from build123d import *

# Parameters (mm, degrees)
F1_DEPTH = 2.25
F2_R     = 0.375
F3_DEPTH = 2.251


with BuildPart() as f1:
    # F0 (on Top) → F1 (new body)
    with BuildSketch(Plane.XY):
        with BuildLine():
            Line((3.396481, 0.154959), (3.496284, 0.161238))
            ThreePointArc((3.496284, 0.161238), (3.474149, 0.424604), (3.432204, 0.685549))
            Line((3.432204, 0.685549), (3.359394, 0.661892))
            Line((3.359394, 0.661892), (3.251238, 0.994762))
            Line((3.251238, 0.994762), (3.346343, 1.025663))
            ThreePointArc((3.346343, 1.025663), (3.259407, 1.27525), (3.153886, 1.517566))
            Line((3.153886, 1.517566), (3.089246, 1.476545))
            Line((3.089246, 1.476545), (2.901707, 1.772059))
            Line((2.901707, 1.772059), (2.98614, 1.825642))
            ThreePointArc((2.98614, 1.825642), (2.839865, 2.045768), (2.677397, 2.254228))
            Line((2.677397, 2.254228), (2.62499, 2.198421))
            Line((2.62499, 2.198421), (2.369851, 2.438012))
            Line((2.369851, 2.438012), (2.438306, 2.510909))
            ThreePointArc((2.438306, 2.510909), (2.241884, 2.687742), (2.032678, 2.849249))
            Line((2.032678, 2.849249), (1.995797, 2.782162))
            Line((1.995797, 2.782162), (1.689089, 2.950775))
            Line((1.689089, 2.950775), (1.737265, 3.038406))
            ThreePointArc((1.737265, 3.038406), (1.503037, 3.160835), (1.260238, 3.265241))
            Line((1.260238, 3.265241), (1.241199, 3.191089))
            Line((1.241199, 3.191089), (0.902195, 3.278131))
            Line((0.902195, 3.278131), (0.927064, 3.374989))
            ThreePointArc((0.927064, 3.374989), (0.669748, 3.435322), (0.408613, 3.476066))
            Line((0.408613, 3.476066), (0.408613, 3.399509))
            Line((0.408613, 3.399509), (0.058613, 3.399509))
            Line((0.058613, 3.399509), (0.058613, 3.499509))
            ThreePointArc((0.058613, 3.499509), (-0.205623, 3.493955), (-0.468687, 3.468477))
            Line((-0.468687, 3.468477), (-0.449648, 3.394325))
            Line((-0.449648, 3.394325), (-0.788652, 3.307284))
            Line((-0.788652, 3.307284), (-0.813521, 3.404142))
            ThreePointArc((-0.813521, 3.404142), (-1.068074, 3.333049), (-1.316537, 3.242951))
            Line((-1.316537, 3.242951), (-1.279656, 3.175864))
            Line((-1.279656, 3.175864), (-1.586363, 3.00725))
            Line((-1.586363, 3.00725), (-1.634538, 3.09488))
            ThreePointArc((-1.634538, 3.09488), (-1.863414, 2.962716), (-2.081665, 2.813658))
            Line((-2.081665, 2.813658), (-2.029258, 2.757851))
            Line((-2.029258, 2.757851), (-2.284397, 2.518259))
            Line((-2.284397, 2.518259), (-2.352852, 2.591156))
            ThreePointArc((-2.352852, 2.591156), (-2.541669, 2.406225), (-2.715994, 2.207573))
            Line((-2.715994, 2.207573), (-2.651355, 2.166552))
            Line((-2.651355, 2.166552), (-2.838894, 1.871037))
            Line((-2.838894, 1.871037), (-2.923327, 1.92462))
            ThreePointArc((-2.923327, 1.92462), (-3.060222, 1.698541), (-3.179667, 1.462778))
            Line((-3.179667, 1.462778), (-3.106857, 1.43912))
            Line((-3.106857, 1.43912), (-3.215013, 1.106251))
            Line((-3.215013, 1.106251), (-3.310119, 1.137152))
            ThreePointArc((-3.310119, 1.137152), (-3.386489, 0.884132), (-3.44355, 0.626071))
            Line((-3.44355, 0.626071), (-3.367144, 0.621264))
            Line((-3.367144, 0.621264), (-3.389121, 0.271954))
            Line((-3.389121, 0.271954), (-3.488923, 0.278234))
            ThreePointArc((-3.488923, 0.278234), (-3.499971, 0.01417), (-3.491062, -0.249974))
            Line((-3.491062, -0.249974), (-3.415861, -0.235629))
            Line((-3.415861, -0.235629), (-3.350278, -0.579429))
            Line((-3.350278, -0.579429), (-3.448506, -0.598168))
            ThreePointArc((-3.448506, -0.598168), (-3.393537, -0.856683), (-3.319218, -1.110313))
            Line((-3.319218, -1.110313), (-3.249947, -1.077716))
            Line((-3.249947, -1.077716), (-3.100924, -1.394406))
            Line((-3.100924, -1.394406), (-3.191407, -1.436984))
            ThreePointArc((-3.191407, -1.436984), (-3.073875, -1.673707), (-2.938815, -1.900886))
            Line((-2.938815, -1.900886), (-2.879827, -1.852087))
            Line((-2.879827, -1.852087), (-2.656728, -2.121766))
            Line((-2.656728, -2.121766), (-2.73378, -2.185509))
            ThreePointArc((-2.73378, -2.185509), (-2.561069, -2.385566), (-2.373755, -2.57202))
            Line((-2.373755, -2.57202), (-2.328756, -2.510084))
            Line((-2.328756, -2.510084), (-2.0456, -2.715809))
            Line((-2.0456, -2.715809), (-2.104379, -2.79671))
            ThreePointArc((-2.104379, -2.79671), (-1.887343, -2.947531), (-1.659544, -3.081544))
            Line((-1.659544, -3.081544), (-1.631362, -3.010363))
            Line((-1.631362, -3.010363), (-1.30594, -3.139207))
            Line((-1.30594, -3.139207), (-1.342752, -3.232184))
            ThreePointArc((-1.342752, -3.232184), (-1.095027, -3.324292), (-0.841058, -3.397443))
            Line((-0.841058, -3.397443), (-0.831463, -3.32149))
            Line((-0.831463, -3.32149), (-0.484223, -3.365357))
            Line((-0.484223, -3.365357), (-0.496756, -3.464568))
            ThreePointArc((-0.496756, -3.464568), (-0.233907, -3.492175), (0.030275, -3.499869))
            Line((0.030275, -3.499869), (0.02068, -3.423916))
            Line((0.02068, -3.423916), (0.36792, -3.380049))
            Line((0.36792, -3.380049), (0.380454, -3.479261))
            ThreePointArc((0.380454, -3.479261), (0.64191, -3.440632), (0.899706, -3.382385))
            Line((0.899706, -3.382385), (0.871524, -3.311204))
            Line((0.871524, -3.311204), (1.196946, -3.182361))
            Line((1.196946, -3.182361), (1.233758, -3.275338))
            ThreePointArc((1.233758, -3.275338), (1.477394, -3.172902), (1.712605, -3.052373))
            Line((1.712605, -3.052373), (1.667606, -2.990438))
            Line((1.667606, -2.990438), (1.950762, -2.784713))
            Line((1.950762, -2.784713), (2.009541, -2.865614))
            ThreePointArc((2.009541, -2.865614), (2.220047, -2.705807), (2.417895, -2.53057))
            Line((2.417895, -2.53057), (2.358907, -2.481771))
            Line((2.358907, -2.481771), (2.582005, -2.212091))
            Line((2.582005, -2.212091), (2.659057, -2.275833))
            ThreePointArc((2.659057, -2.275833), (2.823207, -2.068695), (2.97126, -1.849761))
            Line((2.97126, -1.849761), (2.901989, -1.817165))
            Line((2.901989, -1.817165), (3.051012, -1.500475))
            Line((3.051012, -1.500475), (3.141494, -1.543053))
            ThreePointArc((3.141494, -1.543053), (3.248975, -1.3016), (3.337929, -1.052725))
            Line((3.337929, -1.052725), (3.262728, -1.03838))
            Line((3.262728, -1.03838), (3.328312, -0.69458))
            Line((3.328312, -0.69458), (3.42654, -0.713318))
            ThreePointArc((3.42654, -0.713318), (3.470597, -0.452721), (3.494864, -0.189543))
            Line((3.494864, -0.189543), (3.418458, -0.19435))
            Line((3.418458, -0.19435), (3.396481, 0.154959))
        make_face()
    extrude(amount=F1_DEPTH)

    # F2 (on face) → F3 (cut, through all)
    with BuildSketch(Plane.XY.offset(2.25)):
        Circle(F2_R)
    extrude(amount=-F3_DEPTH, mode=Mode.SUBTRACT)


solid = f1.part
Model file for the job. Use its own axes, mm. Give positions to 0.01 mm unless a question says otherwise; leave off trailing zeros. Loops run counter-clockwise (first coordinate to the right, second up) from the corner with the lowest first, then second, coordinate; pieces in that order, holes last. Notation, with made-up numbers: (-3, -25) -> (17, -25) arc R22 ccw to (17, -12) -> close; hole circle Ø8 at (-12, 66). An arc over 180 degrees is marked (long way). Use a Markdown table: item, result. Add a question column.
(1) Slice it at B-B on x = -0.25. List the corners of the cut face in (y, z), and give its area (3 significant figures).
(2) Slice it at D-D on x = -1.5. List the corners of the cut face in (y, z).
(3) Slice it at C-C on y = -1.25. List the corners of the cut face in (x, z).
(4) Wall check: line 1 along Y through (x, z) = (0.25, 0.6); line 2 along Y through (x, z) = (-1.5, 2); line 3 along X through (y, z) = (2, 0.8). Give the ranges that are in metal, low to high.
(5) Slice it at A-A on y = 0. List the corners of the cut face in (x, z) (3 decimals), and give its area (3 significant figures).
(6) Drop a flat-ended pin along its axis: pin 1 Ø2 at (x, y) = (2, 2) entering from -Z. Give the stop position or say it passes through.
Filled sheet:
| question | item | result |
|---|---|---|
| 1 | outline | (-3.49, 0) -> (-0.28, 0) -> (-0.28, 2.25) -> (-3.49, 2.25) -> close; (0.28, 0) -> (3.49, 0) -> (3.49, 2.25) -> (0.28, 2.25) -> close |
| 1 | area | 14.5 mm2 |
| 2 | outline | (-3.06, 0) -> (3.05, 0) -> (3.05, 2.25) -> (-3.06, 2.25) -> close |
| 3 | outline | (-3.17, 0) -> (3.27, 0) -> (3.27, 2.25) -> (-3.17, 2.25) -> close |
| 4 | line 1 | -3.39 to -0.28, 0.28 to 3.4 |
| 4 | line 2 | -3.06 to 3.05 |
| 4 | line 3 | -2.76 to 2.87 |
| 5 | outline | (-3.5, 0) -> (-0.375, 0) -> (-0.375, 2.25) -> (-3.5, 2.25) -> close; (0.375, 0) -> (3.406, 0) -> (3.406, 2.25) -> (0.375, 2.25) -> close |
| 5 | area | 13.9 mm2 |
| 6 | pin 1 | z = 0 |
